Read the model definition and answer for the solid it produces. Units are mm, in the model's axes. Face numbers are marked on the shaded views. A direction names the side the tool comes from. Round coordinates to 2 decimals unless told otherwise and drop trailing zeros. Write each loop counter-clockwise with the first axis right and the second up, starting at its lowest first coordinate (ties: lowest second). Pieces come first, ordered by that corner, then holes. Notation, with made-up numbers: (-7.75, 61.5) - (23.25, 61.5) arc R14 ccw to (23.25, 87.5) - close; hole circle Ø11 at (-15, 19). An arc over 180 degrees is marked (long way). Use one line per item in the form item = value. Start each with the question number.
1) For a pull along X with two mould halves and no side action, classify the marked faces 5, 6 and 7 as released by +X, released by -X, zero draft, split by the parting line, or undercut.
2) The part is cut by section C-C, the plane y = 2.25. Give the vertices of the cut face in (x, z), plus the area to 3 significant figures.
3) The part is cut by section A-A, the plane z = 6.5. Give the vertices of the cut face in (x, y).
4) Consider line 1 along X through (y, z) = (0.5, 0.5); line 2 along X through (y, z) = (0.5, 1.4); line 3 along Z through (x, y) = (-0.5, 4). Determine where each line is inside the solid, lowest interval first. Write a range as from..to.
5) For the marked faces 1, 2, 3 and 4, determine the directions among +Z, -Z, +X, -X, +Y, -Y from which every point of the face is accessible in a straight line to the end or side of a thin tool.
6) Each of these flat-tipped pins is pushed along its axis until it touches: pin 1 (3.5 mm diameter, centred on x = 0.5, y = 2, fed in from -Z); pin 2 (1 mm diameter, centred on y = 1.5, z = 6, fed in from -X); pin 3 (0.9 mm diameter, centred on x = -5, y = 1.5, fed in from +Z); pin 4 (5 mm diameter, centred on y = -1, z = 10.5, fed in from -X). Where does it stop, or does it pass through?
7) The part is cut by section D-D, the plane z = 9.25. Give the vertices of the cut face in (x, y).
8) The part is cut by section B-B, the plane y = 0.25. Count the separate pieces of the cut face and the enclosed holes in it, plus the area to 3 significant figures.
from build123d import *

# Parameters (mm, degrees)
SKETCH1_W            = 14
SKETCH1_H            = 7
BOSS_EXTRUDE1_DEPTH  = 2
FILLET1_R            = 1.5
M2_CLEARANCE_HOLE1_D = 2.4
SKETCH4_W            = 14
SKETCH4_H            = 12.27377735
BOSS_EXTRUDE2_DEPTH  = 2
BOSS_EXTRUDE3_START  = 1
BOSS_EXTRUDE3_DEPTH  = 1
SKETCH6_W            = 5
SKETCH6_H            = 3.5
CUT_EXTRUDE1_DEPTH   = 1.5
CUT_EXTRUDE2_REACH   = 15.976
SKETCH7_W            = 7
SKETCH7_H            = 2
SKETCH8_W            = 3
SKETCH8_H            = 4
SKETCH8_H_2          = 1
BOSS_EXTRUDE4_DEPTH  = 1.8
CUT_EXTRUDE3_DEPTH   = 2
SKETCH10_W           = 8.1
SKETCH10_H           = 4.09
CUT_EXTRUDE4_DEPTH   = 1
BOSS_EXTRUDE5_DEPTH  = 4.3
SKETCH13_W           = 0.8
SKETCH13_H           = 2.2
CUT_EXTRUDE5_DEPTH   = 5


with BuildPart() as part:
    # Sketch1 → Boss-Extrude1 (new body)
    with BuildSketch(Plane.XY):
        Rectangle(SKETCH1_W, SKETCH1_H)
    extrude(amount=BOSS_EXTRUDE1_DEPTH)

    # Fillet1
    fillet1_edges = [part.edges().sort_by_distance(p)[0] for p in [
        (7, -3.5, 1),
        (-7, -3.5, 1),
    ]]
    fillet(fillet1_edges, radius=FILLET1_R)

    # M2 Clearance Hole1 (through all)
    with Locations(Plane.XY.offset(2)):
        with Locations((-5, 0.5), (5, 0.5)):
            Hole(M2_CLEARANCE_HOLE1_D / 2)

    # Sketch4 → Boss-Extrude2 (add)
    with BuildSketch(Plane(origin=(0, 3.5, 0), x_dir=(1, 0, 0), z_dir=(0, 1, 0))):
        with Locations((0, -6.136888675)):
            Rectangle(SKETCH4_W, SKETCH4_H)
    extrude(amount=BOSS_EXTRUDE2_DEPTH)

    # Sketch5 → Boss-Extrude3 (add)
    with BuildSketch(Plane.XY.offset(2).offset(BOSS_EXTRUDE3_START)):
        with BuildLine():
            ThreePointArc((-7, -2), (-6.560660172, -3.060660172), (-5.5, -3.5))
            Line((-5.5, -3.5), (5.5, -3.5))
            ThreePointArc((5.5, -3.5), (6.560660172, -3.060660172), (7, -2))
            Line((7, -2), (7, 0.5))
            ThreePointArc((7, 0.5), (5.51763809, -1.431851653), (3.267949192, -0.5))
            Line((3.267949192, -0.5), (-3.267949192, -0.5))
            ThreePointArc((-3.267949192, -0.5), (-5.51763809, -1.431851653), (-7, 0.5))
            Line((-7, 0.5), (-7, -2))
        make_face()
    extrude(amount=-BOSS_EXTRUDE3_DEPTH)

    # Sketch6 → Cut-Extrude1 (cut)
    with BuildSketch(Plane(origin=(0, 0, 0), x_dir=(-1, 0, 0), z_dir=(0, 0, -1))):
        with Locations((0, -1.75)):
            Rectangle(SKETCH6_W, SKETCH6_H)
    extrude(amount=-CUT_EXTRUDE1_DEPTH, mode=Mode.SUBTRACT)

    # Sketch7 → Cut-Extrude2 (cut, up to next)
    with BuildSketch(Plane(origin=(0, 0, 1.5), x_dir=(-1, 0, 0), z_dir=(0, 0, -1)), mode=Mode.PRIVATE) as cut_extrude2_sk1:
        with Locations((0, -2.5)):
            Rectangle(SKETCH7_W, SKETCH7_H)
    cut_extrude2_tool1 = extrude(cut_extrude2_sk1.sketch, amount=-CUT_EXTRUDE2_REACH, mode=Mode.PRIVATE) & part.part
    add(cut_extrude2_tool1.solids().sort_by_distance((0, -2.5, 1.5))[0], mode=Mode.SUBTRACT)

    # Sketch8 → Boss-Extrude4 (add)
    with BuildSketch(Plane.XY.offset(2)):
        with Locations((0, 1.5)):
            Rectangle(SKETCH8_W, SKETCH8_H)
        with Locations((0, -1)):
            Rectangle(SKETCH8_W, SKETCH8_H_2)
    extrude(amount=BOSS_EXTRUDE4_DEPTH)

    # Sketch9 → Cut-Extrude3 (cut)
    with BuildSketch(Plane(origin=(0, 5.5, 0), x_dir=(1, 0, 0), z_dir=(0, 1, 0))):
        with BuildLine():
            Line((-2.95, -7.89), (-4.05, -7.89))
            ThreePointArc((-4.05, -7.89), (-4.191421356, -7.831421356), (-4.25, -7.69))
            Line((-4.25, -7.69), (-4.25, -0.83))
            ThreePointArc((-4.25, -0.83), (-4.191421356, -0.688578644), (-4.05, -0.63))
            Line((-4.05, -0.63), (-2.95, -0.63))
            ThreePointArc((-2.95, -0.63), (-2.808578644, -0.688578644), (-2.75, -0.83))
            Line((-2.75, -0.83), (-2.75, -4.1))
            ThreePointArc((-2.75, -4.1), (-2.691421356, -4.241421356), (-2.55, -4.3))
            Line((-2.55, -4.3), (-1.75, -4.3))
            ThreePointArc((-1.75, -4.3), (-1.608578644, -4.358578644), (-1.55, -4.5))
            Line((-1.55, -4.5), (-1.55, -5.5))
            ThreePointArc((-1.55, -5.5), (-1.608578644, -5.641421356), (-1.75, -5.7))
            Line((-1.75, -5.7), (-2.55, -5.7))
            ThreePointArc((-2.55, -5.7), (-2.691421356, -5.758578644), (-2.75, -5.9))
            Line((-2.75, -5.9), (-2.75, -7.69))
            ThreePointArc((-2.75, -7.69), (-2.808578644, -7.831421356), (-2.95, -7.89))
        make_face()
        with BuildLine():
            Line((2.75, -4.1), (2.75, -0.83))
            ThreePointArc((2.75, -0.83), (2.808578644, -0.688578644), (2.95, -0.63))
            Line((2.95, -0.63), (4.05, -0.63))
            ThreePointArc((4.05, -0.63), (4.191421356, -0.688578644), (4.25, -0.83))
            Line((4.25, -0.83), (4.25, -7.69))
            ThreePointArc((4.25, -7.69), (4.191421356, -7.831421356), (4.05, -7.89))
            Line((4.05, -7.89), (2.95, -7.89))
            ThreePointArc((2.95, -7.89), (2.808578644, -7.831421356), (2.75, -7.69))
            Line((2.75, -7.69), (2.75, -5.9))
            ThreePointArc((2.75, -5.9), (2.691421356, -5.758578644), (2.55, -5.7))
            Line((2.55, -5.7), (1.75, -5.7))
            ThreePointArc((1.75, -5.7), (1.608578644, -5.641421356), (1.55, -5.5))
            Line((1.55, -5.5), (1.55, -4.5))
            ThreePointArc((1.55, -4.5), (1.608578644, -4.358578644), (1.75, -4.3))
            Line((1.75, -4.3), (2.55, -4.3))
            ThreePointArc((2.55, -4.3), (2.691421356, -4.241421356), (2.75, -4.1))
        make_face()
    extrude(amount=-CUT_EXTRUDE3_DEPTH, mode=Mode.SUBTRACT)

    # Sketch10 → Cut-Extrude4 (cut)
    with BuildSketch(Plane.XZ.offset(-3.5)):
        with Locations((0, 5.845)):
            Rectangle(SKETCH10_W, SKETCH10_H)
    extrude(amount=-CUT_EXTRUDE4_DEPTH, mode=Mode.SUBTRACT)

    # Sketch12 → Boss-Extrude5 (add)
    with BuildSketch(Plane.XY.offset(12.27377735)):
        with BuildLine():
            Line((7, 3.5), (-7, 3.5))
            ThreePointArc((-7, 3.5), (-6.966992395, 3.345092681), (-6.873703802, 3.217096517))
            ThreePointArc((-6.873703802, 3.217096517), (-6.003119304, 2.685397947), (-5, 2.5))
            ThreePointArc((-5, 2.5), (-3.585786438, 1.914213562), (-3, 0.5))
            ThreePointArc((-3, 0.5), (-3.177124344, -0.322875656), (-3.677124344, -1))
            Line((-3.677124344, -1), (-1.9, -1))
            Line((-1.9, -1), (-1.9, 1.5))
            ThreePointArc((-1.9, 1.5), (0, 3.4), (1.9, 1.5))
            Line((1.9, 1.5), (1.9, -1))
            Line((1.9, -1), (3.677124344, -1))
            ThreePointArc((3.677124344, -1), (3.129171307, 1.207106781), (5, 2.5))
            ThreePointArc((5, 2.5), (6.003119304, 2.685397947), (6.873703802, 3.217096517))
            ThreePointArc((6.873703802, 3.217096517), (6.966992395, 3.345092681), (7, 3.5))
        make_face()
    extrude(amount=-BOSS_EXTRUDE5_DEPTH)

    # Sketch13 → Cut-Extrude5 (cut)
    with BuildSketch(Plane(origin=(0, 3.5, 0), x_dir=(1, 0, 0), z_dir=(0, 1, 0))):
        with Locations((3.53, -1.9)):
            Rectangle(SKETCH13_W, SKETCH13_H)
    cut_extrude5 = extrude(amount=-CUT_EXTRUDE5_DEPTH, mode=Mode.SUBTRACT)

    # Mirror1: Cut-Extrude5 across plane
    add(cut_extrude5.mirror(Plane(origin=(0, 0, 0), x_dir=(0, 0, 1), z_dir=(1, 0, 0))), mode=Mode.SUBTRACT)


solid = part.part
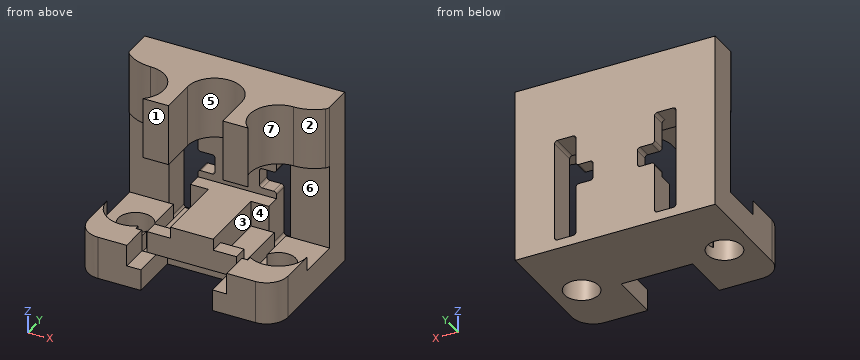
Geometry results:
q1.face_5 = undercut
q1.face_6 = zero draft
q1.face_7 = released by +X
q2.outline = (-7, 0) - (7, 0) - (7, 2) - (3.93, 2) - (3.93, 0.8) - (3.13, 0.8) - (3.13, 2) - (1.5, 2) - (1.5, 3.8) - (-1.5, 3.8) - (-1.5, 2) - (-3.13, 2) - (-3.13, 0.8) - (-3.93, 0.8) - (-3.93, 2) - (-7, 2) - close; (-4.03, 7.97) - (-1.75, 7.97) - (-1.75, 12.27) - (-4.03, 12.27) - close; (1.75, 7.97) - (4.03, 7.97) - (4.03, 12.27) - (1.75, 12.27) - close
q2.area = 51.1 mm2
q3.outline = (-7, 3.5) - (-4.25, 3.5) - (-4.25, 5.5) - (-7, 5.5) - close; (-2.75, 4.5) - (2.75, 4.5) - (2.75, 5.5) - (-2.75, 5.5) - close; (4.25, 3.5) - (7, 3.5) - (7, 5.5) - (4.25, 5.5) - close
q4.line_1 = -7..-6.2, -3.8..3.8, 6.2..7
q4.line_2 = -7..-6.2, -3.13..3.13, 6.2..7
q4.line_3 = 0..3.8, 7.89..12.27
q5.face_1 = +Z, +X, -X, -Y
q5.face_2 = +Z, +X, -Y
q5.face_3 = none
q5.face_4 = +X
q6.pin_1 = 0
q6.pin_2 = through
q6.pin_3 = 2
q6.pin_4 = -3.68
q7.outline = (-7, 3.5) arc R0.38 ccw to (-6.87, 3.22) arc R2.81 ccw to (-5, 2.5) arc R2 cw to (-3.68, -1) - (-1.9, -1) - (-1.9, 1.5) arc R1.9 cw to (1.9, 1.5) - (1.9, -1) - (3.68, -1) arc R2 cw to (5, 2.5) arc R2.81 ccw to (6.87, 3.22) arc R0.38 ccw to (7, 3.5) - (7, 5.5) - (-7, 5.5) - close
q8.separate_pieces = 5
q8.enclosed_holes = 0
q8.area = 32.0 mm2
